Geometry check sheet. Reference: the model listing, model coordinates, mm. A direction names the side the tool comes from. Give positions to 0.01 mm unless a question says otherwise; leave off trailing zeros. Write each loop counter-clockwise with the first axis right and the second up, starting at its lowest first coordinate (ties: lowest second). Pieces come first, ordered by that corner, then holes. Notation, with made-up numbers: (-6.75, -23.75) -> (14.25, -23.75) arc R23 cw to (14.25, 0.25) -> close; hole circle Ø11 at (57.5, -25). An arc over 180 degrees is marked (long way). Use a Markdown table: item, result. Add a question column.
from build123d import *

# Parameters (mm, degrees)
SKETCH_1_W        = 200
SKETCH_1_H        = 135
SKETCH_1_W_2      = 84.112104212
SKETCH_1_H_2      = 90
EXTRUDE_1_DEPTH   = 20
SKETCH_3_R        = 35
SKETCH_3_R_2      = 25
EXTRUDE_1_2_DEPTH = 230
SKETCH_4_R        = 25
EXTRUDE_2_DEPTH   = 50


with BuildPart() as part:
    # Эскиз1 → Extrude 1 (new body)
    with BuildSketch(Plane(origin=(0, 0, 0), x_dir=(1, 0, 0), z_dir=(0, 1, 0))):
        with Locations((45, 0)):
            Rectangle(SKETCH_1_W, SKETCH_1_H)
        with Locations((82.056052106, 0)):
            Rectangle(SKETCH_1_W_2, SKETCH_1_H_2, mode=Mode.SUBTRACT)
    extrude(amount=EXTRUDE_1_DEPTH)

    # Эскиз3 → Extrude 1 2 (add)
    with BuildSketch(Plane(origin=(0, 20, 0), x_dir=(1, 0, 0), z_dir=(0, 1, 0))):
        Circle(SKETCH_3_R)
        Circle(SKETCH_3_R_2, mode=Mode.SUBTRACT)
    extrude(amount=EXTRUDE_1_2_DEPTH)

    # Эскиз4 → Бобышка-Вытянуть2 (add)
    with BuildSketch(Plane(origin=(0, 250, 0), x_dir=(1, 0, 0), z_dir=(0, 1, 0))):
        with BuildLine():
            Line((38.567048096, 27.880540306), (38.567048096, -27.601676263))
            ThreePointArc((38.567048096, -27.601676263), (35.38747425, -34.914800567), (27.87069068, -37.577401116))
            Line((27.87069068, -37.577401116), (-27.024888661, -33.745404507))
            ThreePointArc((-27.024888661, -33.745404507), (-33.641655548, -30.590105807), (-36.328531244, -23.769679653))
            Line((-36.328531244, -23.769679653), (-36.328531244, 23.781195095))
            ThreePointArc((-36.328531244, 23.781195095), (-33.658156001, 30.583885807), (-27.07321106, 33.753429146))
            Line((-27.07321106, 33.753429146), (27.822368281, 37.852774357))
            ThreePointArc((27.822368281, 37.852774357), (35.369738808, 35.210165063), (38.567048096, 27.880540306))
        make_face()
        Circle(SKETCH_4_R, mode=Mode.SUBTRACT)
    extrude(amount=EXTRUDE_2_DEPTH)


solid = part.part
1) Sectioned sample at B-B, the plane x = 51. Enter the section's corners in (y, z).
2) Tool access check on faces 4 (the face through (81, 10, 45)), 5 (the face through (23.846, 158.04, -7.509)), 6 (the face through (-36.329, 275, 0)). Record the directions out of +Z, -Z, +X, -X, +Y, -Y that give a thin tool (end or side, any length) a straight path to the whole face; none if there is none.
3) Sectioned sample at C-C, the plane x = 0. Enter the section's corners in (y, z).
4) Draft check along X on faces 1 (the face through (124.112, 10, 1)), 2 (the face through (44, 10, 67.5)), 3 (the face through (-55, 10, 1)). Enter one of: +X half, -X half, draft (parallel to the pull), parting line (faces both ways), or undercut.
5) Sectioned sample at A-A, the plane z = 0. Enter the section's corners in (x, y), and give its area (3 significant figures).
6) Sectioned sample at D-D, the plane y = 160. Enter the section's corners in (x, z).
7) Gauge pin test, flat ends, axial feed: P1, Ø4, axis at y = 41, z = -25, coming from the +X side; P2, Ø15, axis at y = 285, z = 6, coming from the +X side; P3, Ø4, axis at x = -25, y = 154.5, coming from the +Z side. Record the tip position at first contact, or that the pin passes through.
8) Material ranges on probe 1 along Z at (x, y) = (0, 181); probe 2 along X at (y, z) = (13, 24), recorded low to high. Write a range as [from, to].
Check values:
| question | item | result |
|---|---|---|
| 1 | outline | (0, -67.5) -> (20, -67.5) -> (20, -45) -> (0, -45) -> close; (0, 45) -> (20, 45) -> (20, 67.5) -> (0, 67.5) -> close |
| 2 | face 4 | +Y, -Y |
| 2 | face 5 | +Y |
| 2 | face 6 | +Z, -Z, -X, +Y |
| 3 | outline | (0, -67.5) -> (20, -67.5) -> (20, -35) -> (250, -35) -> (250, -35.78) -> (300, -35.78) -> (300, -25) -> (20, -25) -> (20, 25) -> (300, 25) -> (300, 35.63) -> (250, 35.63) -> (250, 35) -> (20, 35) -> (20, 67.5) -> (0, 67.5) -> close |
| 4 | face 1 | undercut |
| 4 | face 2 | draft |
| 4 | face 3 | -X half |
| 5 | outline | (-55, 0) -> (40, 0) -> (40, 20) -> (35, 20) -> (35, 250) -> (38.57, 250) -> (38.57, 300) -> (25, 300) -> (25, 20) -> (-25, 20) -> (-25, 300) -> (-36.33, 300) -> (-36.33, 250) -> (-35, 250) -> (-35, 20) -> (-55, 20) -> close; (124.11, 0) -> (145, 0) -> (145, 20) -> (124.11, 20) -> close |
| 5 | area | 8,160 mm² |
| 6 | outline | circle Ø70 at (0, 0); hole circle Ø50 at (0, 0) |
| 7 | P1 | x = 26.38 |
| 7 | P2 | x = 38.57 |
| 7 | P3 | z = 26.38 |
| 8 | probe 1 | [-35, -25], [25, 35] |
| 8 | probe 2 | [-55, 40], [124.11, 145] |
